For this review, take the finished solid that the model builds, in its own axes (mm). Round coordinates to 2 decimals unless told otherwise and drop trailing zeros. Order: outer loops, then holes, each group sorted by start corner. A loop starts at its lowest first (then second) coordinate and runs counter-clockwise, first axis right, second up. Notation, with made-up numbers: (86.5, 2) -> (121.5, 2) arc R18 ccw to (121.5, 21) -> close; hole circle Ø3 at (11.5, -34). An arc over 180 degrees is marked (long way). Use a Markdown table: item, result. Add a question column.
1) Wall thickness on line 1 along Y through (x, z) = (0, 3.65); line 2 along Y through (x, z) = (-7.75, 1.5); line 3 along Z through (x, y) = (-0.75, 3.25): over which ranges is each line inside the solid? List them lowest first. Write a range as [from, to].
2) Consider section A-A (y = 0). State the section outline as (x, z) points.
3) Consider section C-C (y = 4). State the section outline as (x, z) points, plus the area to 3 significant figures.
4) Draft analysis for pull direction Y (two halves, no side actions). For faces 1 (the face through (7.52, -3.09, 3.22)), 2 (the face through (-7.61, -5.07, 3.13)), 3 (the face through (7.61, 5.07, 3.13)), 4 (the face through (-5.7, -5.8, 3.2)), state which applies: pulls with the +Y half, pulls with the -Y half, needs draft (parallel to the pull), parting line crosses it, or undercut.
5) Clearance check with flat-ended pins moving along their axes: P1, Ø1, axis at x = -4.5, z = 5.5, coming from the -Y side; P2, Ø1, axis at x = 4, z = 2.5, coming from the +Y side; P3, Ø2, axis at y = 5, z = 2, coming from the -X side. State where each tip first meets the part, or that it passes through.
```python
from build123d import *

# Parameters (mm, degrees)
F0_R     = 9.144
F1_DEPTH = 6.35
F2_R     = 1.5621
F3_DEPTH = 6.351
F4_SIZE2 = 1.244969
F4_SIZE  = 1.778
F5_R     = 1.016
F6_DEPTH = 6.351


with BuildPart() as f1:
    # F0 (on Top) → F1 (new body)
    with BuildSketch(Plane.XY):
        Circle(F0_R)
    extrude(amount=F1_DEPTH)

    # F2 (on face) → F3 (cut, through all)
    with BuildSketch(Plane.XY.offset(6.35)):
        Circle(F2_R)
    extrude(amount=-F3_DEPTH, mode=Mode.SUBTRACT)

    # F4
    f4_edges = [f1.edges().sort_by_distance(p)[0] for p in [
        (-1.5621, 0, 0),
    ]]
    chamfer(f4_edges, length=F4_SIZE, length2=F4_SIZE2)

    # F5 (on face) → F6 (cut, through all)
    with BuildSketch(Plane.XY.offset(6.35)):
        with BuildLine():
            ThreePointArc((0, 8.128), (0.71842, 8.42558), (1.016, 9.144))
            ThreePointArc((1.016, 9.144), (-0.71842, 9.86242), (0, 8.128))
        make_face()
        with Locations((-3.499257, 8.447954)):
            Circle(F5_R)
        with Locations((-6.465784, 6.465784)):
            Circle(F5_R)
        with Locations((-8.447954, 3.499257)):
            Circle(F5_R)
        with Locations((-9.144, 0)):
            Circle(F5_R)
        with Locations((-8.447954, -3.499257)):
            Circle(F5_R)
        with Locations((-6.465784, -6.465784)):
            Circle(F5_R)
        with Locations((-3.499257, -8.447954)):
            Circle(F5_R)
        with Locations((0, -9.144)):
            Circle(F5_R)
        with Locations((3.499257, -8.447954)):
            Circle(F5_R)
        with Locations((6.465784, -6.465784)):
            Circle(F5_R)
        with Locations((8.447954, -3.499257)):
            Circle(F5_R)
        with Locations((9.144, 0)):
            Circle(F5_R)
        with Locations((8.447954, 3.499257)):
            Circle(F5_R)
        with Locations((6.465784, 6.465784)):
            Circle(F5_R)
        with Locations((3.499257, 8.447954)):
            Circle(F5_R)
    extrude(amount=-F6_DEPTH, mode=Mode.SUBTRACT)


solid = f1.part
```
Results list:
| question | item | result |
|---|---|---|
| 1 | line 1 | [-8.13, -1.56], [1.56, 8.13] |
| 1 | line 2 | [-4.85, -4.24], [-2.76, 2.76], [4.24, 4.85] |
| 1 | line 3 | [0, 6.35] |
| 2 | outline | (-8.13, 0) -> (-3.34, 0) -> (-1.56, 1.24) -> (-1.56, 6.35) -> (-8.13, 6.35) -> close; (1.56, 1.24) -> (3.34, 0) -> (8.13, 0) -> (8.13, 6.35) -> (1.56, 6.35) -> close |
| 3 | outline | (-7.56, 0) -> (7.56, 0) -> (7.56, 6.35) -> (-7.56, 6.35) -> close |
| 3 | area | 96.1 mm2 |
| 4 | face 1 | undercut |
| 4 | face 2 | pulls with the -Y half |
| 4 | face 3 | pulls with the +Y half |
| 4 | face 4 | undercut |
| 5 | P1 | y = -8.01 |
| 5 | P2 | y = 8.01 |
| 5 | P3 | x = -8.01 |
